```python
from build123d import *

# Parameters (mm, degrees)
SKETCH1_R           = 1
BOSS_EXTRUDE1_DEPTH = 3.3
CUT_EXTRUDE1_START  = -1
SKETCH2_R           = 1
CUT_EXTRUDE1_DEPTH  = 1


with BuildPart() as part:
    # Sketch1 → Boss-Extrude1 (new body)
    with BuildSketch(Plane.XY):
        with BuildLine():
            Line((-47.825, -19.975), (-47.825, -23.875))
            ThreePointArc((-47.825, -23.875), (-46.082285348, -28.082285348), (-41.875, -29.825))
            Line((-41.875, -29.825), (-40.475, -29.825))
            ThreePointArc((-40.475, -29.825), (-39.520405845, -29.429594155), (-39.125, -28.475))
            Line((-39.125, -28.475), (-39.125, -22.044366415))
            ThreePointArc((-39.125, -22.044366415), (-39.375745502, -21.260695854), (-40.034836368, -20.768139171))
            Line((-40.034836368, -20.768139171), (-46.034836368, -18.698772757))
            ThreePointArc((-46.034836368, -18.698772757), (-47.258670561, -18.875745502), (-47.825, -19.975))
        make_face()
        with Locations((-45, -24)):
            Circle(SKETCH1_R, mode=Mode.SUBTRACT)
    extrude(amount=BOSS_EXTRUDE1_DEPTH)

    # Sketch2 → Cut-Extrude1 (cut)
    with BuildSketch(Plane.XY.offset(3.3).offset(CUT_EXTRUDE1_START)):
        with BuildLine():
            Line((-40.263069362, -21.429886631), (-46.263069362, -19.360520216))
            ThreePointArc((-46.263069362, -19.360520216), (-46.852322863, -19.445729316), (-47.125, -19.975))
            Line((-47.125, -19.975), (-47.125, -23.875))
            ThreePointArc((-47.125, -23.875), (-45.587310601, -27.587310601), (-41.875, -29.125))
            Line((-41.875, -29.125), (-40.475, -29.125))
            ThreePointArc((-40.475, -29.125), (-40.015380592, -28.934619408), (-39.825, -28.475))
            Line((-39.825, -28.475), (-39.825, -22.044366415))
            ThreePointArc((-39.825, -22.044366415), (-39.945729316, -21.667043552), (-40.263069362, -21.429886631))
        make_face()
        with Locations((-45, -24)):
            Circle(SKETCH2_R, mode=Mode.SUBTRACT)
    extrude(amount=CUT_EXTRUDE1_DEPTH, mode=Mode.SUBTRACT)


solid = part.part
```
The listing builds one solid part. Answer for the finished solid, in the listing's coordinates (mm). A direction names the side the tool comes from. Round coordinates to 2 decimals unless told otherwise and drop trailing zeros. Order: outer loops, then holes, each group sorted by start corner. A loop starts at its lowest first (then second) coordinate and runs counter-clockwise, first axis right, second up. Notation, with made-up numbers: (-35, -6) -> (19, -6) arc R16 cw to (19, 0) -> close; hole circle Ø4 at (-13, 51.25). An arc over 180 degrees is marked (long way). Answer as CSV lines item,"result". Start each with the question number.
(1) The part is cut by section D-D (y = -25.75). Determine the outline of the cut face in (x, z) (3 decimals).
(2) The part is cut by section A-A (y = -23.75). Determine the outline of the cut face in (x, z) (3 decimals), then the cut area to 3 significant figures.
(3) For a pull along X with two mould halves and no side action, classify faces 3 (the face through (-42.99, -19.75, 1.63)), 4 (the face through (-46.845, -19.441, 2.793)), 5 (the face through (-47.4, -24.2, 3.3)) as +X half, -X half, draft (parallel to the pull), parting line (faces both ways), or undercut.
(4) A tool of negligible diameter and unlimited length cuts with its end or side. For faces 1 (the face through (-43.22, -20.41, 2.79)), 2 (the face through (-39.125, -25, 2)), from which of +Z, -Z, +X, -X, +Y, -Y can it reach the whole face along a straight path? Write none if from no direction.
(5) Find the intervals of material crossed by probe 1 along Z at (x, y) = (-43.5, -22.5); probe 2 along Y at (x, z) = (-40.5, 2.55) (3 decimals); probe 3 along X at (y, z) = (-25.25, 2.7) (3 decimals), in increasing order. Write a range as from..to.
(6) The part is cut by section B-B (x = -45.5). Determine the outline of the cut face in (y, z), then the cut area to 3 significant figures.
(7) The part is cut by section C-C (x = -40.75). Determine the outline of the cut face in (y, z) (3 decimals).
(8) Flat-ended cylindrical pins translate along their axes: pin 1 Ø1 at (x, y) = (-45.5, -22.5) entering from +Z; pin 2 Ø1.5 at (y, z) = (-21, 2) entering from +X; pin 3 Ø0.8 at (x, z) = (-41, 3) entering from +Y. Find the tip coordinate at first contact, or state that the pin passes through.
Evaluation:
1,outline,"(-47.522, 0) -> (-39.125, 0) -> (-39.125, 3.3) -> (-39.825, 3.3) -> (-39.825, 2.3) -> (-46.779, 2.3) -> (-46.779, 3.3) -> (-47.522, 3.3) -> close"
2,outline,"(-47.825, 0) -> (-45.968, 0) -> (-45.968, 2.3) -> (-47.125, 2.3) -> (-47.125, 3.3) -> (-47.825, 3.3) -> close; (-44.032, 0) -> (-39.125, 0) -> (-39.125, 3.3) -> (-39.825, 3.3) -> (-39.825, 2.3) -> (-44.032, 2.3) -> close"
2,area,"17.0 mm²"
3,face 3,"+X half"
3,face 4,"undercut"
3,face 5,"draft"
4,face 1,"+Z"
4,face 2,"+Z, -Z, +X, +Y, -Y"
5,probe 1,"0..2.3"
5,probe 2,"-29.825..-29.125, -21.348..-20.608"
5,probe 3,"-47.664..-46.942, -39.825..-39.125"
6,outline,"(-28.59, 0) -> (-24.87, 0) -> (-24.87, 2.3) -> (-27.67, 2.3) -> (-27.67, 3.3) -> (-28.59, 3.3) -> close; (-23.13, 0) -> (-18.88, 0) -> (-18.88, 3.3) -> (-19.62, 3.3) -> (-19.62, 2.3) -> (-23.13, 2.3) -> close"
6,area,"20.0 mm²"
7,outline,"(-29.825, 0) -> (-20.521, 0) -> (-20.521, 3.3) -> (-21.262, 3.3) -> (-21.262, 2.3) -> (-29.125, 2.3) -> (-29.125, 3.3) -> (-29.825, 3.3) -> close"
8,pin 1,"z = 2.3"
8,pin 2,"x = -39.16"
8,pin 3,"y = -20.3"
